from build123d import *

# Parameters (mm, degrees)
BOSS_EXTRUDE1_DEPTH  = 3
SKETCH3_R            = 1.35
CUT_EXTRUDE1_DEPTH   = 4
SKETCH4_W            = 6
SKETCH4_H            = 27
BOSS_EXTRUDE2_DEPTH  = 32
SKETCH5_R            = 9
CUT_EXTRUDE2_DEPTH   = 29
SKETCH6_W            = 8
SKETCH6_H            = 25
CUT_EXTRUDE3_DEPTH   = 3
SKETCH7_R            = 2.5
SKETCH7_R_2          = 1.65
BOSS_EXTRUDE3_DEPTH  = 3
SKETCH8_R            = 1.65
CUT_EXTRUDE4_DEPTH   = 3
CHAMFER1_SIZE        = 0.6
SKETCH9_R            = 2.75
CUT_EXTRUDE5_DEPTH   = 1
CHAMFER2_SIZE        = 3
CHAMFER3_SIZE        = 3
SKETCH10_W           = 32
SKETCH10_H           = 27
CUT_EXTRUDE6_DEPTH   = 20
SKETCH11_R           = 1.65
BOSS_EXTRUDE5_DEPTH  = 3
BOSS_EXTRUDE6_DEPTH  = 3
SKETCH12_R           = 9
BOSS_EXTRUDE7_DEPTH  = 3
SKETCH15_W           = 25.06
SKETCH15_H           = 26.2
CUT_EXTRUDE7_DEPTH   = 4
SKETCH16_W           = 12.8
SKETCH16_H           = 12.8
CUT_EXTRUDE8_DEPTH   = 3
SKETCH17_W           = 12.16
SKETCH17_H           = 4.8
SKETCH17_W_2         = 4.4
BOSS_EXTRUDE8_DEPTH  = 3
SKETCH18_R           = 1.15
CUT_EXTRUDE9_DEPTH   = 6
SKETCH19_R           = 2
CUT_EXTRUDE11_DEPTH  = 1.8
CUT_EXTRUDE13_DEPTH  = 0.2
SKETCH21_W           = 2.3
SKETCH21_H           = 2.3
CUT_EXTRUDE14_DEPTH  = 0.2
CHAMFER4_SIZE        = 0.6
SKETCH22_W           = 1.4
SKETCH22_H           = 26.2
CUT_EXTRUDE15_DEPTH  = 4
BOSS_EXTRUDE9_DEPTH  = 32
SKETCH24_W           = 8.54
SKETCH24_H           = 16.6
CUT_EXTRUDE16_DEPTH  = 1
BOSS_EXTRUDE10_DEPTH = 2
CHAMFER5_SIZE        = 1


with BuildPart() as part:
    # Sketch2 → Boss-Extrude1 (new body)
    with BuildSketch(Plane.XY):
        Polygon((-65, 21.5), (-37, 21.5), (-37, 13.5), (-59, 13.5), (-59, -13.5), (-37, -13.5), (-37, -21.5), (-65, -21.5), align=None)
    extrude(amount=BOSS_EXTRUDE1_DEPTH)

    # Sketch3 → Cut-Extrude1 (cut, through all)
    with BuildSketch(Plane.XY.offset(3)):
        with Locations((-41, 17.5)):
            Circle(SKETCH3_R)
        with Locations((-61, 17.5)):
            Circle(SKETCH3_R)
        with Locations((-61, -17.5)):
            Circle(SKETCH3_R)
        with Locations((-41, -17.5)):
            Circle(SKETCH3_R)
    extrude(amount=-CUT_EXTRUDE1_DEPTH, mode=Mode.SUBTRACT)

    # Sketch4 → Boss-Extrude2 (add)
    with BuildSketch(Plane.XY.offset(3)):
        with Locations((-62, 0)):
            Rectangle(SKETCH4_W, SKETCH4_H)
    extrude(amount=BOSS_EXTRUDE2_DEPTH)

    # Sketch5 → Cut-Extrude2 (cut, through all)
    with BuildSketch(Plane.ZY.offset(65)):
        with Locations((23, 0)):
            Circle(SKETCH5_R)
    extrude(amount=-CUT_EXTRUDE2_DEPTH, mode=Mode.SUBTRACT)

    # Sketch6 → Cut-Extrude3 (cut)
    with BuildSketch(Plane(origin=(-59, 0, 0), x_dir=(0, 0, -1), z_dir=(1, 0, 0))):
        with Locations((-23, 0)):
            Rectangle(SKETCH6_W, SKETCH6_H)
    extrude(amount=-CUT_EXTRUDE3_DEPTH, mode=Mode.SUBTRACT)

    # Sketch7 → Boss-Extrude3 (add)
    with BuildSketch(Plane(origin=(-59, 0, 0), x_dir=(0, 0, -1), z_dir=(1, 0, 0))):
        with Locations((-30, 10.5)):
            Circle(SKETCH7_R)
        with Locations((-30, 10.5)):
            Circle(SKETCH7_R_2, mode=Mode.SUBTRACT)
        with Locations((-16, 10.5)):
            Circle(SKETCH7_R)
        with Locations((-16, 10.5)):
            Circle(SKETCH7_R_2, mode=Mode.SUBTRACT)
        with Locations((-16, -10.5)):
            Circle(SKETCH7_R)
        with Locations((-16, -10.5)):
            Circle(SKETCH7_R_2, mode=Mode.SUBTRACT)
        with Locations((-30, -10.5)):
            Circle(SKETCH7_R)
        with Locations((-30, -10.5)):
            Circle(SKETCH7_R_2, mode=Mode.SUBTRACT)
    extrude(amount=BOSS_EXTRUDE3_DEPTH)

    # Sketch8 → Cut-Extrude4 (cut)
    with BuildSketch(Plane(origin=(-59, 0, 0), x_dir=(0, 0, -1), z_dir=(1, 0, 0))):
        with Locations((-30, -10.5)):
            Circle(SKETCH8_R)
        with Locations((-16, -10.5)):
            Circle(SKETCH8_R)
        with Locations((-16, 10.5)):
            Circle(SKETCH8_R)
        with Locations((-30, 10.5)):
            Circle(SKETCH8_R)
    extrude(amount=-CUT_EXTRUDE4_DEPTH, mode=Mode.SUBTRACT)

    # Chamfer1
    chamfer1_edges = [part.edges().sort_by_distance(p)[0] for p in [
        (-65, 13.5, 19),
        (-65, -13.5, 19),
    ]]
    chamfer(chamfer1_edges, length=CHAMFER1_SIZE)

    # Sketch9 → Cut-Extrude5 (cut)
    with BuildSketch(Plane.XY.offset(3)):
        with Locations((-61, 17.5)):
            Circle(SKETCH9_R)
        with Locations((-41, 17.5)):
            Circle(SKETCH9_R)
        with Locations((-41, -17.5)):
            Circle(SKETCH9_R)
        with Locations((-61, -17.5)):
            Circle(SKETCH9_R)
    extrude(amount=-CUT_EXTRUDE5_DEPTH, mode=Mode.SUBTRACT)

    # Chamfer2
    chamfer2_edges = [part.edges().sort_by_distance(p)[0] for p in [
        (-59, 13.5, 1.5),
        (-59, -13.5, 1.5),
    ]]
    chamfer(chamfer2_edges, length=CHAMFER2_SIZE)

    # Chamfer3
    chamfer3_edges = [part.edges().sort_by_distance(p)[0] for p in [
        (-65, 21.5, 1.5),
        (-65, -21.5, 1.5),
    ]]
    chamfer(chamfer3_edges, length=CHAMFER3_SIZE)

    # Sketch10 → Cut-Extrude6 (cut)
    with BuildSketch(Plane(origin=(-59, 0, 0), x_dir=(0, 0, -1), z_dir=(1, 0, 0))):
        with Locations((-19, 0)):
            Rectangle(SKETCH10_W, SKETCH10_H)
    extrude(amount=CUT_EXTRUDE6_DEPTH, mode=Mode.SUBTRACT)

    # Sketch11 → Boss-Extrude5 (add)
    with BuildSketch(Plane(origin=(-59, 0, 0), x_dir=(0, 0, -1), z_dir=(1, 0, 0))):
        with Locations((-30, 10.5)):
            Circle(SKETCH11_R)
        with Locations((-16, 10.5)):
            Circle(SKETCH11_R)
        with Locations((-16, -10.5)):
            Circle(SKETCH11_R)
        with Locations((-30, -10.5)):
            Circle(SKETCH11_R)
    extrude(amount=-BOSS_EXTRUDE5_DEPTH)

    # Sketch11<3> → Boss-Extrude6 (add)
    with BuildSketch(Plane(origin=(-59, 0, 0), x_dir=(0, 0, -1), z_dir=(1, 0, 0))):
        with BuildLine():
            ThreePointArc((-27, 8.062257748), (-32, 0), (-27, -8.062257748))
            Line((-27, -8.062257748), (-27, -12.5))
            Line((-27, -12.5), (-19, -12.5))
            Line((-19, -12.5), (-19, -8.062257748))
            ThreePointArc((-19, -8.062257748), (-14, 0), (-19, 8.062257748))
            Line((-19, 8.062257748), (-19, 12.5))
            Line((-19, 12.5), (-27, 12.5))
            Line((-27, 12.5), (-27, 8.062257748))
        make_face()
    extrude(amount=-BOSS_EXTRUDE6_DEPTH)

    # Sketch12 → Boss-Extrude7 (add)
    with BuildSketch(Plane.ZY.offset(62)):
        with Locations((23, 0)):
            Circle(SKETCH12_R)
    extrude(amount=BOSS_EXTRUDE7_DEPTH)

    # Sketch15 → Cut-Extrude7 (cut)
    with BuildSketch(Plane(origin=(-59, 0, 0), x_dir=(0, 0, -1), z_dir=(1, 0, 0))):
        with Locations((-21.07, 0)):
            Rectangle(SKETCH15_W, SKETCH15_H)
    extrude(amount=-CUT_EXTRUDE7_DEPTH, mode=Mode.SUBTRACT)

    # Sketch16 → Cut-Extrude8 (cut, through all)
    with BuildSketch(Plane(origin=(-63, 0, 0), x_dir=(0, 0, -1), z_dir=(1, 0, 0))):
        with Locations((-18.6, 0)):
            Rectangle(SKETCH16_W, SKETCH16_H)
    extrude(amount=-CUT_EXTRUDE8_DEPTH, mode=Mode.SUBTRACT)

    # Sketch17 → Boss-Extrude8 (add)
    with BuildSketch(Plane(origin=(-63, 0, 0), x_dir=(0, 0, -1), z_dir=(1, 0, 0))):
        with Locations((-14.62, -10.7)):
            Rectangle(SKETCH17_W, SKETCH17_H)
        with Locations((-31, -10.7)):
            Rectangle(SKETCH17_W_2, SKETCH17_H)
        with Locations((-31, 10.7)):
            Rectangle(SKETCH17_W_2, SKETCH17_H)
        with Locations((-14.62, 10.7)):
            Rectangle(SKETCH17_W, SKETCH17_H)
    extrude(amount=BOSS_EXTRUDE8_DEPTH)

    # Sketch18 → Cut-Extrude9 (cut, through all)
    with BuildSketch(Plane(origin=(-60, 0, 0), x_dir=(0, 0, -1), z_dir=(1, 0, 0))):
        with Locations((-31, 10.5)):
            Circle(SKETCH18_R)
        with Locations((-18.5, 10.5)):
            Circle(SKETCH18_R)
        with Locations((-18.5, -10.5)):
            Circle(SKETCH18_R)
        with Locations((-31, -10.5)):
            Circle(SKETCH18_R)
    extrude(amount=-CUT_EXTRUDE9_DEPTH, mode=Mode.SUBTRACT)

    # Sketch19 → Cut-Extrude11 (cut)
    with BuildSketch(Plane.ZY.offset(65)):
        with Locations((18.5, 10.5)):
            Circle(SKETCH19_R)
        with Locations((31, 10.5)):
            Circle(SKETCH19_R)
        with Locations((31, -10.5)):
            Circle(SKETCH19_R)
        with Locations((18.5, -10.5)):
            Circle(SKETCH19_R)
    extrude(amount=-CUT_EXTRUDE11_DEPTH, mode=Mode.SUBTRACT)

    # Sketch20 → Cut-Extrude13 (cut)
    with BuildSketch(Plane.ZY.offset(63.2)):
        with BuildLine():
            Line((17.35, 8.863693183), (17.35, 12.136306817))
            ThreePointArc((17.35, 12.136306817), (18.5, 12.5), (19.65, 12.136306817))
            Line((19.65, 12.136306817), (19.65, 8.863693183))
            ThreePointArc((19.65, 8.863693183), (18.5, 8.5), (17.35, 8.863693183))
        make_face()
        with BuildLine():
            Line((29.85, 8.863693183), (29.85, 12.136306817))
            ThreePointArc((29.85, 12.136306817), (31, 12.5), (32.15, 12.136306817))
            Line((32.15, 12.136306817), (32.15, 8.863693183))
            ThreePointArc((32.15, 8.863693183), (31, 8.5), (29.85, 8.863693183))
        make_face()
    cut_extrude13 = extrude(amount=-CUT_EXTRUDE13_DEPTH, mode=Mode.SUBTRACT)

    # Sketch21 → Cut-Extrude14 (cut)
    with BuildSketch(Plane.ZY.offset(63)):
        with Locations((18.5, 10.5)):
            Rectangle(SKETCH21_W, SKETCH21_H)
        with Locations((31, 10.5)):
            Rectangle(SKETCH21_W, SKETCH21_H)
    cut_extrude14 = extrude(amount=-CUT_EXTRUDE14_DEPTH, mode=Mode.SUBTRACT)

    # Mirror1: Cut-Extrude13, Cut-Extrude14 across plane
    add(cut_extrude13.mirror(Plane.ZX), mode=Mode.SUBTRACT)
    add(cut_extrude14.mirror(Plane.ZX), mode=Mode.SUBTRACT)

    # Chamfer4
    chamfer4_edges = [part.edges().sort_by_distance(p)[0] for p in [
        (-65, 0, 25),
        (-65, 6.4, 18.6),
        (-65, 0, 12.2),
        (-65, -6.4, 18.6),
    ]]
    chamfer(chamfer4_edges, length=CHAMFER4_SIZE)

    # Sketch22 → Cut-Extrude15 (cut)
    with BuildSketch(Plane(origin=(-59, 0, 0), x_dir=(0, 0, -1), z_dir=(1, 0, 0))):
        with Locations((-34.3, 0)):
            Rectangle(SKETCH22_W, SKETCH22_H)
    extrude(amount=-CUT_EXTRUDE15_DEPTH, mode=Mode.SUBTRACT)

    # Sketch23 → Boss-Extrude9 (add)
    with BuildSketch(Plane.XY.offset(35)):
        Polygon((-64.4, 13.5), (-63.4, 14.5), (-59, 14.5), (-59, 13.5), align=None)
        Polygon((-59, -13.5), (-64.4, -13.5), (-63.4, -14.5), (-59, -14.5), align=None)
    extrude(amount=-BOSS_EXTRUDE9_DEPTH)

    # Sketch24 → Cut-Extrude16 (cut)
    with BuildSketch(Plane(origin=(-59, 0, 0), x_dir=(0, 0, -1), z_dir=(1, 0, 0))):
        with Locations((-4.27, 0)):
            Rectangle(SKETCH24_W, SKETCH24_H)
    extrude(amount=-CUT_EXTRUDE16_DEPTH, mode=Mode.SUBTRACT)

    # Sketch27 → Boss-Extrude10 (add)
    with BuildSketch(Plane.XY.offset(35)):
        Polygon((-59, 14.5), (-63.4, 14.5), (-65, 12.9), (-65, -12.9), (-63.4, -14.5), (-59, -14.5), align=None)
    extrude(amount=BOSS_EXTRUDE10_DEPTH)

    # Chamfer5
    chamfer5_edges = [part.edges().sort_by_distance(p)[0] for p in [
        (-65, 0, 37),
    ]]
    chamfer(chamfer5_edges, length=CHAMFER5_SIZE)


solid = part.part
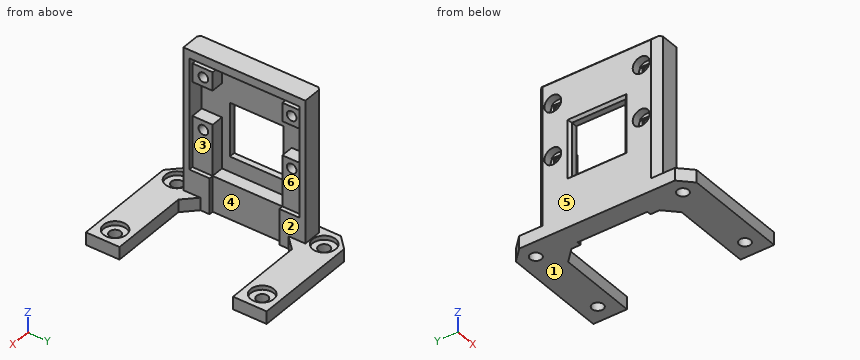
Geometry check sheet. Reference: the model listing, model coordinates, mm. Face numbers are marked on the shaded views. A direction names the side the tool comes from. Round coordinates to 2 decimals unless told otherwise and drop trailing zeros. Loops run counter-clockwise (first coordinate to the right, second up) from the corner with the lowest first, then second, coordinate; pieces in that order, holes last. Notation, with made-up numbers: (-37, -0.5) -> (-15, -0.5) arc R16 ccw to (-15, 13.5) -> close; hole circle Ø5 at (-24.5, 25.25). An arc over 180 degrees is marked (long way). Answer as a JSON object with one key per item and string values. Group by question number.
Item 1: Cross-section at A-A, the plane y = 17.5. Record the cut outline in (x, z).
Item 2: Thickness scan on line 1 along Y through (x, z) = (-61, 2.5); line 2 along Y through (x, z) = (-41, 2.3); line 3 along Y through (x, z) = (-60.6, 31). Record the ranges inside material, lowest first.
Item 3: Cross-section at B-B, the plane x = -50.5. Record the cut outline in (y, z), plus the area to 3 significant figures.
Item 4: Set-up check for the marked faces 4, 5 and 6: record each of +Z, -Z, +X, -X, +Y, -Y from which the full face is reachable in a straight line by a thin tool's end or side.
Item 5: Release check for a two-part mould opening along Z. For the marked faces 1, 2 and 3 record: pulls with the +Z half, pulls with the -Z half, needs draft (parallel to the pull), parting line crosses it, or undercut.
Item 6: Depth check by flat-ended pin: pin 1 Ø5 at (x, y) = (-41, 17.5) entering from +Z; pin 2 Ø3.5 at (x, z) = (-61.5, 32) entering from -Y; pin 3 Ø3.5 at (y, z) = (12, 31) entering from +X. Enter the tip coordinate at first touch or a pass-through.
Item 7: Cross-section at C-C, the plane y = 0. Record the cut outline in (x, z), plus the area to 3 significant figures.
Item 8: Cross-section at D-D, the plane z = 6. Record the cut outline in (x, y).
Determined:
{
 "1": {"outline": "(-65, 0) -> (-62.35, 0) -> (-62.35, 2) -> (-63.75, 2) -> (-63.75, 3) -> (-65, 3) -> close; (-59.65, 0) -> (-42.35, 0) -> (-42.35, 2) -> (-43.75, 2) -> (-43.75, 3) -> (-58.25, 3) -> (-58.25, 2) -> (-59.65, 2) -> close; (-39.65, 0) -> (-37, 0) -> (-37, 3) -> (-38.25, 3) -> (-38.25, 2) -> (-39.65, 2) -> close"},
 "2": {"line 1": "y = -21.5 to -20.25, -14.75 to 14.75, 20.25 to 21.5", "line 2": "y = -21.5 to -20.25, -14.75 to -13.5, 13.5 to 14.75, 20.25 to 21.5", "line 3": "y = -14.5 to -11.65, -9.35 to -8.3, 8.3 to 9.35, 11.65 to 14.5"},
 "3": {"outline": "(-21.5, 0) -> (-13.5, 0) -> (-13.5, 3) -> (-21.5, 3) -> close; (13.5, 0) -> (21.5, 0) -> (21.5, 3) -> (13.5, 3) -> close", "area": "48.0 mm²"},
 "4": {"face 4": "-Z, +X", "face 5": "+Z, -Z, -X, +Y, -Y", "face 6": "+X"},
 "5": {"face 1": "pulls with the -Z half", "face 2": "needs draft", "face 3": "undercut"},
 "6": {"pin 1": "stops at z = 2", "pin 2": "stops at y = -14.5", "pin 3": "stops at x = -59"},
 "7": {"outline": "(-65, 0) -> (-60, 0) -> (-60, 8.54) -> (-63, 8.54) -> (-63, 12.2) -> (-64.4, 12.2) -> (-65, 11.6) -> close; (-65, 25.6) -> (-64.4, 25) -> (-63, 25) -> (-63, 35) -> (-59, 35) -> (-59, 37) -> (-64, 37) -> (-65, 36) -> close", "area": "81.2 mm²"},
 "8": {"outline": "(-65, -12.9) -> (-63.4, -14.5) -> (-59, -14.5) -> (-59, -8.3) -> (-60, -8.3) -> (-60, 8.3) -> (-59, 8.3) -> (-59, 14.5) -> (-63.4, 14.5) -> (-65, 12.9) -> close"}
}
